Build history of the part. All positions in model axes, mm. A direction names the side the tool comes from. Give positions to 0.01 mm unless a question says otherwise; leave off trailing zeros. Order: outer loops, then holes, each group sorted by start corner. A loop starts at its lowest first (then second) coordinate and runs counter-clockwise, first axis right, second up. Notation, with made-up numbers: M 38,68.25 L 69,68.25 A24 cw 69,85.25 Z; hole C -36,76 d2. An arc over 180 degrees is marked long. One line per item, written item: value.
from build123d import *

# Parameters (mm, degrees)
BOSS_EXTRUDE1_DEPTH = 4
SKETCH3_R           = 2
CUT_EXTRUDE1_DEPTH  = 10
CUT_EXTRUDE2_DEPTH  = 10
SKETCH5_W           = 37.5
SKETCH5_H           = 5
SKETCH5_R           = 2
CUT_EXTRUDE3_DEPTH  = 10
SKETCH6_R           = 2
CUT_EXTRUDE4_DEPTH  = 10
SKETCH7_R           = 1
CUT_EXTRUDE5_DEPTH  = 10
SKETCH8_R           = 2
CUT_EXTRUDE6_DEPTH  = 10


with BuildPart() as part:
    # Sketch1 → Boss-Extrude1 (new body)
    # profile 1 of 2: a face of its own
    with BuildSketch(Plane.XY):
        with BuildLine():
            Line((0, -57.20543624), (0, 140.79456376))
            Line((0, 140.79456376), (-50, 140.79456376))
            Line((-50, 140.79456376), (-65.293896859, 140.79456376))
            ThreePointArc((-65.293896859, 140.79456376), (-83.510437362, 132.343917874), (-88.822955159, 112.978151212))
            ThreePointArc((-88.822955159, 112.978151212), (-82.121571276, 106.62300147), (-74.161000128, 111.305498795))
            Line((-74.161000128, 111.305498795), (-70.965431907, 118.996456291))
            ThreePointArc((-70.965431907, 118.996456291), (-68.695430494, 121.757834263), (-65.274420897, 122.79456376))
            Line((-65.274420897, 122.79456376), (-50.707299907, 122.79456376))
            Line((-50.707299907, 122.79456376), (-42.5, 122.79456376))
            ThreePointArc((-42.5, 122.79456376), (-38.964466094, 121.330097666), (-37.5, 117.79456376))
            Line((-37.5, 117.79456376), (-37.5, 95.998067584))
            Line((-37.5, 95.998067584), (-85, 22.344598664))
            Line((-85, 22.344598664), (-85, -51.456618505))
            Line((-85, -51.456618505), (-76.438195827, -57.20543624))
            Line((-76.438195827, -57.20543624), (0, -57.20543624))
        make_face()
        with BuildLine():
            ThreePointArc((-37.5, 27.79456376), (-38.964466094, 24.259029854), (-42.5, 22.79456376))
            Line((-42.5, 22.79456376), (-74.161000128, 22.79456376))
            Line((-74.161000128, 22.79456376), (-37.5, 79.641086571))
            Line((-37.5, 79.641086571), (-37.5, 27.79456376))
        make_face(mode=Mode.SUBTRACT)
    # profile 2 of 2: a face of its own
    with BuildSketch(Plane.XY):
        with BuildLine():
            Line((65.293896859, 140.79456376), (50, 140.79456376))
            Line((50, 140.79456376), (0, 140.79456376))
            Line((0, 140.79456376), (0, -57.20543624))
            Line((0, -57.20543624), (76.438195827, -57.20543624))
            Line((76.438195827, -57.20543624), (85, -51.456618505))
            Line((85, -51.456618505), (85, 22.344598664))
            Line((85, 22.344598664), (37.5, 95.998067584))
            Line((37.5, 95.998067584), (37.5, 117.79456376))
            ThreePointArc((37.5, 117.79456376), (38.964466094, 121.330097666), (42.5, 122.79456376))
            Line((42.5, 122.79456376), (50.707299907, 122.79456376))
            Line((50.707299907, 122.79456376), (65.274420897, 122.79456376))
            ThreePointArc((65.274420897, 122.79456376), (68.695430494, 121.757834263), (70.965431907, 118.996456291))
            Line((70.965431907, 118.996456291), (74.161000128, 111.305498795))
            ThreePointArc((74.161000128, 111.305498795), (82.121571276, 106.62300147), (88.822955159, 112.978151212))
            ThreePointArc((88.822955159, 112.978151212), (83.510437362, 132.343917874), (65.293896859, 140.79456376))
        make_face()
        with BuildLine():
            Line((37.5, 79.641086571), (74.161000128, 22.79456376))
            Line((74.161000128, 22.79456376), (42.5, 22.79456376))
            ThreePointArc((42.5, 22.79456376), (38.964466094, 24.259029854), (37.5, 27.79456376))
            Line((37.5, 27.79456376), (37.5, 79.641086571))
        make_face(mode=Mode.SUBTRACT)
    extrude(amount=BOSS_EXTRUDE1_DEPTH)

    # Sketch3 → Cut-Extrude1 (cut)
    with BuildSketch(Plane.XY.offset(4)):
        with Locations((-47.324700565, 132.53476761)):
            Circle(SKETCH3_R)
        with Locations((47.324700565, 132.53476761)):
            Circle(SKETCH3_R)
    extrude(amount=-CUT_EXTRUDE1_DEPTH, mode=Mode.SUBTRACT)

    # Sketch4 → Cut-Extrude2 (cut)
    with BuildSketch(Plane.XY.offset(4)):
        with BuildLine():
            Line((-99.472025614, 6.792585345), (-83.380037388, 6.792585345))
            ThreePointArc((-83.380037388, 6.792585345), (-81.258717044, 5.913905689), (-80.380037388, 3.792585345))
            Line((-80.380037388, 3.792585345), (-80.380037388, -41.949469703))
            ThreePointArc((-80.380037388, -41.949469703), (-81.258717044, -44.070790047), (-83.380037388, -44.949469703))
            Line((-83.380037388, -44.949469703), (-99.472025614, -44.949469703))
            Line((-99.472025614, -44.949469703), (-99.472025614, 6.792585345))
        make_face()
        with BuildLine():
            Line((99.472025614, -44.949469703), (83.380037388, -44.949469703))
            ThreePointArc((83.380037388, -44.949469703), (81.258717044, -44.070790047), (80.380037388, -41.949469703))
            Line((80.380037388, -41.949469703), (80.380037388, 3.792585345))
            ThreePointArc((80.380037388, 3.792585345), (81.258717044, 5.913905689), (83.380037388, 6.792585345))
            Line((83.380037388, 6.792585345), (99.472025614, 6.792585345))
            Line((99.472025614, 6.792585345), (99.472025614, -44.949469703))
        make_face()
    extrude(amount=-CUT_EXTRUDE2_DEPTH, mode=Mode.SUBTRACT)

    # Sketch5 → Cut-Extrude3 (cut)
    with BuildSketch(Plane.XY.offset(4)):
        with Locations((-18.75, 132.551936771)):
            Rectangle(SKETCH5_W, SKETCH5_H)
        with Locations((18.75, 132.551936771)):
            Rectangle(SKETCH5_W, SKETCH5_H)
        with Locations((20, 112.567697597)):
            Circle(SKETCH5_R)
        with Locations((-20, 112.567697597)):
            Circle(SKETCH5_R)
    extrude(amount=-CUT_EXTRUDE3_DEPTH, mode=Mode.SUBTRACT)

    # Sketch6 → Cut-Extrude4 (cut)
    with BuildSketch(Plane.XY.offset(4)):
        with Locations((28.728783517, 5.096950375)):
            Circle(SKETCH6_R)
        with Locations((69.728783517, -35.903049625)):
            Circle(SKETCH6_R)
    extrude(amount=-CUT_EXTRUDE4_DEPTH, mode=Mode.SUBTRACT)

    # Sketch7 → Cut-Extrude5 (cut)
    with BuildSketch(Plane.XY.offset(4)):
        with Locations((-76.177192192, -14.107414655)):
            Circle(SKETCH7_R)
        with Locations((-76.177192192, -24.107414655)):
            Circle(SKETCH7_R)
        with Locations((76.177192192, -24.107414655)):
            Circle(SKETCH7_R)
        with Locations((76.177192192, -14.107414655)):
            Circle(SKETCH7_R)
    extrude(amount=-CUT_EXTRUDE5_DEPTH, mode=Mode.SUBTRACT)

    # Sketch8 → Cut-Extrude6 (cut)
    with BuildSketch(Plane.XY.offset(4)):
        with Locations((-27.6, -48.199469703)):
            Circle(SKETCH8_R)
        with Locations((31.57, -48.199469703)):
            Circle(SKETCH8_R)
    extrude(amount=-CUT_EXTRUDE6_DEPTH, mode=Mode.SUBTRACT)


solid = part.part
1) Saw through at B-B, the plane y = 75.5. Write the cut outline in (x, z).
Check values:
outline: M -50.72,0 L -40.17,0 L -40.17,4 L -50.72,4 Z; M -37.5,0 L 37.5,0 L 37.5,4 L -37.5,4 Z; M 40.17,0 L 50.72,0 L 50.72,4 L 40.17,4 Z
2) Tool access for faces 1 (the face through (-60.918, 59.687, 1.972)), 2 (the face through (55.57, 51.62, 1.97)), 3 (the face through (1, 140.795, 2)): list every direction of +Z, -Z, +X, -X, +Y, -Y with a clear straight run to the whole face (end or side of a thin tool).
Check values:
face 1: +Z, -Z, -X
face 2: +Z, -Z
face 3: +Z, -Z, +X, -X, +Y
3) Pin check, flat tips, straight feed: pin 1 (0.5 mm diameter, centred on x = 84, z = 2, fed in from -Y); pin 2 (1.5 mm diameter, centred on y = -24.5, z = 1, fed in from +X); pin 3 (1.2 mm diameter, centred on y = 133, z = 1.5, fed in from +X). Stop position of each tip, or through.
Check values:
pin 1: y = -52.3
pin 2: x = 80.38
pin 3: x = 83.46
4) Mould opens along X. For faces 4 (the face through (-80.38, -19, 2)), 5 (the face through (-18.92, 114.25, 2.03)), 6 (the face through (83.7, 132.12, 1.97)), 7 (the face through (37.5, 53, 2)) say: released by +X, released by -X, zero draft, split by the parting line, or undercut.
Check values:
face 4: released by -X
face 5: undercut
face 6: released by +X
face 7: undercut
5) Saw through at D-D, the plane y = -1.5. Write the cut outline in (x, z).
Check values:
outline: M -80.38,0 L 80.38,0 L 80.38,4 L -80.38,4 Z
6) Drill centre lines: probe 1 along X at (y, z) = (-24, 1.35); probe 2 along Y at (x, z) = (20, 1.4); probe 3 along Y at (x, z) = (-27.6, 3). Where is each one in solid material? Low to high. Write a range as from..to.
Check values:
probe 1: -80.38..-77.17, -75.18..75.18, 77.17..80.38
probe 2: -57.21..110.57, 114.57..130.05, 135.05..140.79
probe 3: -57.21..-50.2, -46.2..130.05, 135.05..140.79
7) Saw through at C-C, the plane x = -60.5. Write the cut outline in (y, z), then the cut area to 3 significant figures.
Check values:
outline: M -57.21,0 L 22.79,0 L 22.79,4 L -57.21,4 Z; M 43.98,0 L 60.33,0 L 60.33,4 L 43.98,4 Z; M 122.79,0 L 140.79,0 L 140.79,4 L 122.79,4 Z
area: 457 mm^2
8) Saw through at A-A, the plane x = -15. Write the cut outline in (y, z), then the cut area to 3 significant figures.
Check values:
outline: M -57.21,0 L 130.05,0 L 130.05,4 L -57.21,4 Z; M 135.05,0 L 140.79,0 L 140.79,4 L 135.05,4 Z
area: 772 mm^2
